Check sheet for the drawn part. Datum: minimum x, y, z corner. Units: mm. A direction names the side the tool comes from. Round coordinates to 2 decimals unless told otherwise and drop trailing zeros. Write each loop counter-clockwise with the first axis right and the second up, starting at its lowest first coordinate (ties: lowest second). Pieces come first, ordered by that corner, then holes. Notation, with made-up numbers: M -29.75,60 L -0.75,60 A28 cw -0.75,78 Z; hole C -33,-6 d7. An arc over 180 degrees is marked long. One line per item, written item: value. Start each with the question number.
Item 1: Gauge pin test, flat ends, axial feed: pin 1 (24 mm diameter, centred on y = 67.5, z = 39, fed in from +X); pin 2 (6 mm diameter, centred on x = 34.5, y = 30, fed in from +Z); pin 3 (6 mm diameter, centred on x = 14.5, z = 7, fed in from +Y); pin 4 (2 mm diameter, centred on y = 35, z = 23, fed in from -X). Record the tip position at first contact, or that the pin passes through.
Item 2: Section check B-B, the plane z = 17. Record the cut outline in (x, y), then the cut area to 3 significant figures.
Item 3: Section check A-A, the plane x = 10.5. Record the cut outline in (y, z), then the cut area to 3 significant figures.
Item 4: Tool access check on the marked faces 1, 2 and 3. Record the directions out of +Z, -Z, +X, -X, +Y, -Y that give a thin tool (end or side, any length) a straight path to the whole face; none if there is none.
Item 5: Section check C-C, the plane y = 91. Record the cut outline in (x, z).
Item 6: Thickness scan on probe 1 along Y at (x, z) = (28, 8); probe 2 along X at (y, z) = (35, 37.5); probe 3 along Z at (x, y) = (7.5, 130.5). Record the ranges inside material, lowest first. Write a range as from..to.
Item 7: Section check D-D, the plane z = 25. Record the cut outline in (x, y).
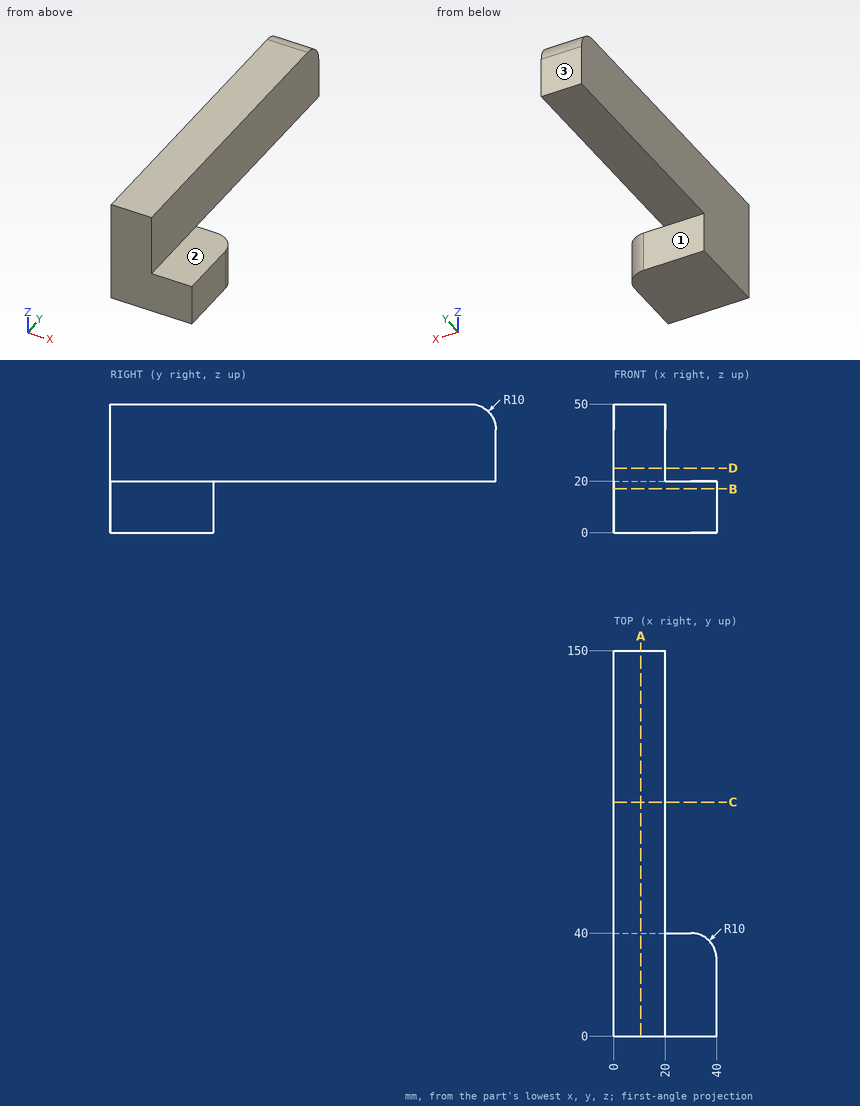
Response values:
1. pin 1: stops at x = 20
1. pin 2: stops at z = 20
1. pin 3: stops at y = 40
1. pin 4: stops at x = 0
2. outline: M 0,0 L 40,0 L 40,30 A10 ccw 30,40 L 0,40 Z
2. area: 1,580 mm2
3. outline: M 0,0 L 40,0 L 40,20 L 150,20 L 150,40 A10 ccw 140,50 L 0,50 Z
3. area: 5,280 mm2
4. face 1: -Z, +X, -X, +Y
4. face 2: +Z, +X, +Y, -Y
4. face 3: +Z, -Z, +X, -X, +Y
5. outline: M 0,20 L 20,20 L 20,50 L 0,50 Z
6. probe 1: y = 0..40
6. probe 2: x = 0..20
6. probe 3: z = 20..50
7. outline: M 0,0 L 20,0 L 20,150 L 0,150 Z
